```python
from build123d import *

# Parameters (mm, degrees)
SKETCH1_R           = 2.5
BOSS_EXTRUDE1_DEPTH = 3.175
FILLET1_R           = 2


with BuildPart() as part:
    # Sketch1 → Boss-Extrude1 (new body)
    with BuildSketch(Plane.XY):
        Polygon((-20, 20), (20, 20), (20, -20), (30.352761804, -58.637033052), (-6.967746272, -68.637033052), (-20, -20), align=None)
        with Locations((-15, 15)):
            Circle(SKETCH1_R, mode=Mode.SUBTRACT)
        with Locations((-15, -15)):
            Circle(SKETCH1_R, mode=Mode.SUBTRACT)
        with Locations((15, 15)):
            Circle(SKETCH1_R, mode=Mode.SUBTRACT)
        with Locations((15, -15)):
            Circle(SKETCH1_R, mode=Mode.SUBTRACT)
        with Locations((-11.855046207, -33.711914808)):
            Circle(SKETCH1_R, mode=Mode.SUBTRACT)
        with Locations((17.122728582, -25.947343455)):
            Circle(SKETCH1_R, mode=Mode.SUBTRACT)
        with Locations((24.887299935, -54.925118244)):
            Circle(SKETCH1_R, mode=Mode.SUBTRACT)
        with Locations((-4.090474854, -62.689689597)):
            Circle(SKETCH1_R, mode=Mode.SUBTRACT)
        Polygon((10.823922003, 0), (7.653668647, 7.653668647), (0, 10.823922003), (-7.653668647, 7.653668647), (-10.823922003, 0), (-7.653668647, -7.653668647), (0, -10.823922003), (7.653668647, -7.653668647), align=None, mode=Mode.SUBTRACT)
    extrude(amount=BOSS_EXTRUDE1_DEPTH)

    # Fillet1
    fillet1_edges = [part.edges().sort_by_distance(p)[0] for p in [
        (-20, 20, 1.5875),
        (20, 20, 1.5875),
        (20, -20, 1.5875),
        (30.352761804, -58.637033052, 1.5875),
        (-6.967746272, -68.637033052, 1.5875),
        (-20, -20, 1.5875),
    ]]
    fillet(fillet1_edges, radius=FILLET1_R)


solid = part.part
```
Design review of the part built by this model. Coordinates are the model's own, in mm. A direction names the side the tool comes from. Coordinates: 2 decimals unless noted, no trailing zeros. Order: outer loops, then holes, each group sorted by start corner. A loop starts at its lowest first (then second) coordinate and runs counter-clockwise, first axis right, second up. Notation, with made-up numbers: (61.5, 46) -> (67.5, 46) arc R31 ccw to (67.5, 72) -> close; hole circle Ø6 at (-18.75, -35.75). An arc over 180 degrees is marked (long way). One line per item, written item: value. Start each with the question number.
Q1. Mouldability with a two-part tool opening along X and no side actions: class faces 1 (the cylindrical face through (-6.57, -67.91, 1.61)), 2 (the flat face through (20, -1, 2)), 3 (the flat face through (9.261, 3.773, 1.565)) as pulls with the +X half, pulls with the -X half, needs draft (parallel to the pull), parting line crosses it, or undercut.
Q2. Take a section at A-A, the plane y = -15. State the section outline as (x, z) points (3 decimals).
Q3. Tool access review of faces 4 (the flat face through (9.217, -3.88, 1.565)), 5 (the flat face through (-20, -1, 2)): name each direction out of +Z, -Z, +X, -X, +Y, -Y from which nothing blocks a thin tool from reaching the whole face with its end or side.
Q4. Take a section at B-B, the plane x = 6.5. State the section outline as (y, z) points (3 decimals), then the cut area to 3 significant figures.
Q5. For probe 1 along Y at (x, z) = (-4, 2.2); probe 2 along Y at (x, z) = (16, 1.1); probe 3 along Y at (x, z) = (-3, 1.75), list the stretches that pass through material, from the lowest coordinate up.
Q6. Take a section at C-C, the plane z = 1.2. Give the number of separate pieces and of enclosed holes in the cut face, then the cut area to 3 significant figures.
Q7. Take a section at D-D, the plane x = -3.5. State the section outline as (y, z) points (3 decimals).
Values follow:
1. face 1: parting line crosses it
1. face 2: pulls with the +X half
1. face 3: undercut
2. outline: (-20, 0) -> (-17.5, 0) -> (-17.5, 3.175) -> (-20, 3.175) -> close; (-12.5, 0) -> (12.5, 0) -> (12.5, 3.175) -> (-12.5, 3.175) -> close; (17.5, 0) -> (20, 0) -> (20, 3.175) -> (17.5, 3.175) -> close
3. face 4: +Z, -Z
3. face 5: +Z, -Z, -X, +Y, -Y
4. outline: (-65.028, 0) -> (-8.132, 0) -> (-8.132, 3.175) -> (-65.028, 3.175) -> close; (8.132, 0) -> (20, 0) -> (20, 3.175) -> (8.132, 3.175) -> close
4. area: 218 mm2
5. probe 1: y = -67.84 to -65.19, -60.19 to -9.17, 9.17 to 20
5. probe 2: y = -62.48 to -28.18, -23.71 to -17.29, -12.71 to 12.71, 17.29 to 20
5. probe 3: y = -67.57 to -64.94, -60.44 to -9.58, 9.58 to 20
6. separate pieces: 1
6. enclosed holes: 9
6. area: 2,850 mm2
7. outline: (-67.708, 0) -> (-65.119, 0) -> (-65.119, 3.175) -> (-67.708, 3.175) -> close; (-60.26, 0) -> (-9.374, 0) -> (-9.374, 3.175) -> (-60.26, 3.175) -> close; (9.374, 0) -> (20, 0) -> (20, 3.175) -> (9.374, 3.175) -> close
